```python
from build123d import *

# Parameters (mm, degrees)
F0_W      = 127
F0_H      = 0.1285925341
F0_H_2    = 228.4714074659
F0_W_2    = 15.24
F0_H_3    = 19.05
F3_DEPTH  = 6.35
F2_W      = 31.75
F2_H      = 31.75
F4_DEPTH  = 12.7
F5_W      = 36.83
F5_H      = 66.039527216
F6_DEPTH  = 50.8
F7_R      = 1.27
F8_DEPTH  = 12.7
F9_R      = 4.445
F10_DEPTH = 12.7


with BuildPart() as f3:
    # F0 (on Front) → F3 (new body, symmetric)
    with BuildSketch(Plane.XZ):
        Polygon((-63.5, 114.1714074659), (-63.5, 114.3), (63.5, 114.3), (63.5, 114.1714074659), (69.85, 114.1714074659), (69.85, 129.4114074659), (63.5, 129.4114074659), (-63.5, 129.4114074659), (-69.85, 129.4114074659), (-69.85, 114.1714074659), align=None)
        with Locations((0, 114.235703733)):
            Rectangle(F0_W, F0_H)
        with Locations((0, -0.064296267)):
            Rectangle(F0_W, F0_H_2)
        Polygon((63.5, -114.3), (-63.5, -114.3), (-69.85, -114.3), (-69.85, -120.65), (69.85, -120.65), (69.85, -114.3), align=None)
        Polygon((-63.5, 135.7614074659), (-63.5, 129.4114074659), (63.5, 129.4114074659), (63.5, 135.7614074659), (57.15, 135.7614074659), (-57.15, 135.7614074659), align=None)
        Polygon((-57.15, 142.1114074659), (-57.15, 135.7614074659), (57.15, 135.7614074659), (57.15, 142.1114074659), (7.62, 142.1114074659), (-7.62, 142.1114074659), align=None)
        with Locations((0, 151.6364074659)):
            Rectangle(F0_W_2, F0_H_3)
        with BuildLine():
            ThreePointArc((7.62, 161.1614074659), (0, 168.7814074659), (-7.62, 161.1614074659))
            Line((-7.62, 161.1614074659), (7.62, 161.1614074659))
        make_face()
    extrude(amount=F3_DEPTH, both=True)

    # F2 (on face) → F4 (join)
    with BuildSketch(Plane.XZ):
        with Locations((24.2836736143, 87.9182294011)):
            Rectangle(F2_W, F2_H)
    extrude(amount=F4_DEPTH)

    # F5 (on face) → F6 (cut)
    with BuildSketch(Plane.XZ.offset(6.35)):
        with Locations((24.765, 0.0003129244)):
            Rectangle(F5_W, F5_H)
        with Locations((-24.765, 0.0003129244)):
            Rectangle(F5_W, F5_H)
    extrude(amount=-F6_DEPTH, mode=Mode.SUBTRACT)

    # F7 (on face) → F8 (cut, symmetric)
    with BuildSketch(Plane.XZ.offset(6.35)):
        with Locations((-42.0314632356, 100.0508442521)):
            Circle(F7_R)
        with Locations((-6.9654858671, 100.0512316823)):
            Circle(F7_R)
    extrude(amount=F8_DEPTH, both=True, mode=Mode.SUBTRACT)

    # F9 (on face) → F10 (cut, symmetric)
    with BuildSketch(Plane.XZ.offset(6.35)):
        with Locations((-25.4, 52.5126196444)):
            Circle(F9_R)
        with Locations((25.4, 52.5126196444)):
            Circle(F9_R)
        with Locations((-25.4, -52.5126196444)):
            Circle(F9_R)
        with Locations((25.4, -52.5126196444)):
            Circle(F9_R)
    extrude(amount=F10_DEPTH, both=True, mode=Mode.SUBTRACT)


solid = f3.part
```
Here's how the part is built. I have some questions about the finished solid (model axes, mm). A direction names the side the tool comes from. Coordinates: 2 decimals unless noted, no trailing zeros. Order: outer loops, then holes, each group sorted by start corner. A loop starts at its lowest first (then second) coordinate and runs counter-clockwise, first axis right, second up.
Item 1: If we section it at D-D, the plane y = -1: Give the number of separate pieces and of enclosed holes in the cut face, then the cut area to 3 significant figures.
Response values:
separate pieces: 1
enclosed holes: 8
area: 28,800 mm2
Item 2: If we section it at B-B, the plane z = 3.5: List the corners of the cut face in (x, y) for me.
Response values:
outline: (-63.5, -6.35) - (-43.18, -6.35) - (-43.18, 6.35) - (-63.5, 6.35) - close; (-6.35, -6.35) - (6.35, -6.35) - (6.35, 6.35) - (-6.35, 6.35) - close; (43.18, -6.35) - (63.5, -6.35) - (63.5, 6.35) - (43.18, 6.35) - close
Item 3: If we section it at A-A, the plane x = -25.4: List the corners of the cut face in (y, z) for me, then the cut area to 3 significant figures.
Response values:
outline: (-6.35, -120.65) - (6.35, -120.65) - (6.35, -56.96) - (-6.35, -56.96) - close; (-6.35, -48.07) - (6.35, -48.07) - (6.35, -33.02) - (-6.35, -33.02) - close; (-6.35, 33.02) - (6.35, 33.02) - (6.35, 48.07) - (-6.35, 48.07) - close; (-6.35, 56.96) - (6.35, 56.96) - (6.35, 142.11) - (-6.35, 142.11) - close
area: 2,270 mm2
Item 4: Which directions (+Z, -Z, +X, -X, +Y, -Y) give clear straight access to the entire face, cutting with the end or side of a thin tool? Please do faces 4 (the face through (67, 0, -114.3)), 5 (the face through (-67, 0, 114.171)), 6 (the face through (25, 0, 33.02)), 7 (the face through (67, 0, 129.411)).
Response values:
face 4: +X, +Y, -Y
face 5: -X, +Y, -Y
face 6: +Y, -Y
face 7: +Z, +X, +Y, -Y
Item 5: If we section it at C-C, the plane x = 25.4: List the corners of the cut face in (y, z) for me.
Response values:
outline: (-12.7, 72.04) - (-6.35, 72.04) - (-6.35, 56.96) - (6.35, 56.96) - (6.35, 142.11) - (-6.35, 142.11) - (-6.35, 103.79) - (-12.7, 103.79) - close; (-6.35, -120.65) - (6.35, -120.65) - (6.35, -56.96) - (-6.35, -56.96) - close; (-6.35, -48.07) - (6.35, -48.07) - (6.35, -33.02) - (-6.35, -33.02) - close; (-6.35, 33.02) - (6.35, 33.02) - (6.35, 48.07) - (-6.35, 48.07) - close
Item 6: Thinking about a two-plate mould opening in Z: for faces 1 (the face through (24, -9, 103.793)), 2 (the face through (-69.85, 0, -117)), 3 (the face through (63.5, 0, -2)), which applies, pulls with the +Z half, pulls with the -Z half, needs draft (parallel to the pull), parting line crosses it, or undercut?
Response values:
face 1: pulls with the +Z half
face 2: needs draft
face 3: undercut
Item 7: I'm going to push flat-ended pins straight in: pin 1 Ø3 at (x, y) = (18.5, -9) entering from +Z; pin 2 Ø7 at (x, y) = (66.5, 3) entering from +Z; pin 3 Ø6 at (y, z) = (-2, 34) entering from -X. Where does each tip first touch, or does it pass through?
Response values:
pin 1: stops at z = 103.79
pin 2: stops at z = 135.76
pin 3: stops at x = -63.5
Item 8: I need wall thicknesses on probe 1 along Z at (x, y) = (25.4, -2.75); probe 2 along X at (y, z) = (0.5, 20); probe 3 along Z at (x, y) = (-17.5, 0.75). Which ranges of each line are inside material? Lowest first, please.
Response values:
probe 1: z = -120.65 to -56.96, -48.07 to -33.02, 33.02 to 48.07, 56.96 to 142.11
probe 2: x = -63.5 to -43.18, -6.35 to 6.35, 43.18 to 63.5
probe 3: z = -120.65 to -33.02, 33.02 to 142.11
